Geometry check sheet. Reference: the model listing, model coordinates, mm. Face numbers are marked on the shaded views. A direction names the side the tool comes from. Coordinates: 2 decimals unless noted, no trailing zeros. Write each loop counter-clockwise with the first axis right and the second up, starting at its lowest first coordinate (ties: lowest second). Pieces come first, ordered by that corner, then holes. Notation, with made-up numbers: M -10.75,28.25 L -4.75,28.25 A28 ccw -4.75,57.25 Z; hole C 78,47 d6. An arc over 180 degrees is marked long. Write item = value, one per line. Start each with the question number.
```python
from build123d import *

# Parameters (mm, degrees)
BOSS_EXTRUDE1_DEPTH              = 503.65
TOPHOLES_SKETCH2_R               = 12
TOPHOLES_SKETCH2_R_2             = 1.5875
TOPHOLES_CUT_EXTRUDE1_DEPTH      = 507.693115332
BACKSIDEHOLES_SKETCH3_R          = 1.5875
BACKSIDEHOLES_CUT_EXTRUDE2_DEPTH = 507.842305357


with BuildPart() as part:
    # Sketch1 → Boss-Extrude1 (new body)
    with BuildSketch(Plane(origin=(0, 0, 0), x_dir=(0, 0, -1), z_dir=(1, 0, 0))):
        Polygon((0, 0), (-50.8, 0), (-50.8, 3.175), (-3.175, 3.175), (-3.175, 25.4), (0, 25.4), align=None)
    extrude(amount=BOSS_EXTRUDE1_DEPTH)

    # TopHoles-Sketch2 → TopHoles-Cut-Extrude1 (cut, through all)
    with BuildSketch(Plane(origin=(0, 3.175, 0), x_dir=(1, 0, 0), z_dir=(0, 1, 0))):
        with Locations(Location((26.25, -29.8, 0), (0, 0, 270))):
            Circle(TOPHOLES_SKETCH2_R)
        with Locations(Location((477.4, -29.8, 0), (0, 0, 270))):
            Circle(TOPHOLES_SKETCH2_R)
        with Locations(Location((10.75, -14.3, 0), (0, 0, 270))):
            Circle(TOPHOLES_SKETCH2_R_2)
        with Locations(Location((41.75, -14.3, 0), (0, 0, 270))):
            Circle(TOPHOLES_SKETCH2_R_2)
        with Locations(Location((461.9, -14.3, 0), (0, 0, 270))):
            Circle(TOPHOLES_SKETCH2_R_2)
        with Locations(Location((492.9, -14.3, 0), (0, 0, 270))):
            Circle(TOPHOLES_SKETCH2_R_2)
        with Locations(Location((10.75, -45.3, 0), (0, 0, 270))):
            Circle(TOPHOLES_SKETCH2_R_2)
        with Locations(Location((41.75, -45.3, 0), (0, 0, 270))):
            Circle(TOPHOLES_SKETCH2_R_2)
        with Locations(Location((461.9, -45.3, 0), (0, 0, 270))):
            Circle(TOPHOLES_SKETCH2_R_2)
        with Locations(Location((492.9, -45.3, 0), (0, 0, 270))):
            Circle(TOPHOLES_SKETCH2_R_2)
    extrude(amount=-TOPHOLES_CUT_EXTRUDE1_DEPTH, mode=Mode.SUBTRACT)

    # BackSideHoles-Sketch3 → BackSideHoles-Cut-Extrude2 (cut, through all)
    with BuildSketch(Plane(origin=(0, 0, 0), x_dir=(-1, 0, 0), z_dir=(0, 0, -1))):
        with Locations(Location((-495.7125, 17.4625, 0), (0, 0, 90))):
            Circle(BACKSIDEHOLES_SKETCH3_R)
        with Locations(Location((-486.1875, 17.4625, 0), (0, 0, 90))):
            Circle(BACKSIDEHOLES_SKETCH3_R)
        with Locations(Location((-490.95, 11.1125, 0), (0, 0, 90))):
            Circle(BACKSIDEHOLES_SKETCH3_R)
        with Locations(Location((-12.7, 11.1125, 0), (0, 0, 90))):
            Circle(BACKSIDEHOLES_SKETCH3_R)
        with Locations(Location((-17.4625, 17.4625, 0), (0, 0, 90))):
            Circle(BACKSIDEHOLES_SKETCH3_R)
        with Locations(Location((-7.9375, 17.4625, 0), (0, 0, 90))):
            Circle(BACKSIDEHOLES_SKETCH3_R)
    extrude(amount=-BACKSIDEHOLES_CUT_EXTRUDE2_DEPTH, mode=Mode.SUBTRACT)


solid = part.part
```
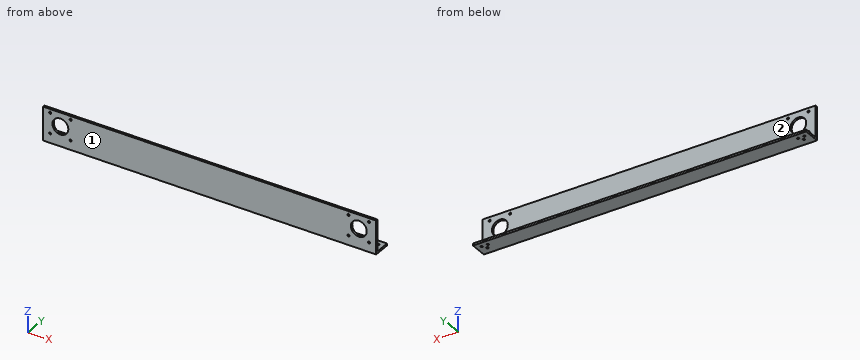
Q1. Cross-section at B-B on x = 284. Enter the section's corners in (y, z) (3 decimals), and give its area (3 significant figures).
Q2. Cross-section at A-A on z = 29.8. Enter the section's corners in (x, y) (3 decimals), and give its area (3 significant figures).
Q3. Set-up check for the marked faces 1 and 2: record each of +Z, -Z, +X, -X, +Y, -Y from which the full face is reachable in a straight line by a thin tool's end or side.
Q4. Scan lines: L1, parallel to X at y = 1.9, z = 14.3; L2, parallel to Z at x = 273, y = 7.5 (3 decimals). Record each from-to range of solid material in increasing order.
Q5. Gauge pin test, flat ends, axial feed: pin 1 (10 mm diameter, centred on x = 255, y = 23, fed in from -Z); pin 2 (10 mm diameter, centred on x = 402.5, z = 21, fed in from +Y) (3 decimals). Record the tip position at first contact, or that the pin passes through.
Values found:
q1.outline = M 0,0 L 25.4,0 L 25.4,3.175 L 3.175,3.175 L 3.175,50.8 L 0,50.8 Z
q1.area = 232 mm²
q2.outline = M 0,0 L 14.25,0 L 14.25,3.175 L 0,3.175 Z; M 38.25,0 L 465.4,0 L 465.4,3.175 L 38.25,3.175 Z; M 489.4,0 L 503.65,0 L 503.65,3.175 L 489.4,3.175 Z
q2.area = 1,450 mm²
q3.face_1 = +Z, -Z, +X, -X, -Y
q3.face_2 = +Z, +X, -X, +Y
q4.L1 = 0 to 9.16, 12.34 to 40.16, 43.34 to 460.31, 463.49 to 491.31, 494.49 to 503.65
q4.L2 = 0 to 3.175
q5.pin_1 = 0
q5.pin_2 = 3.175
